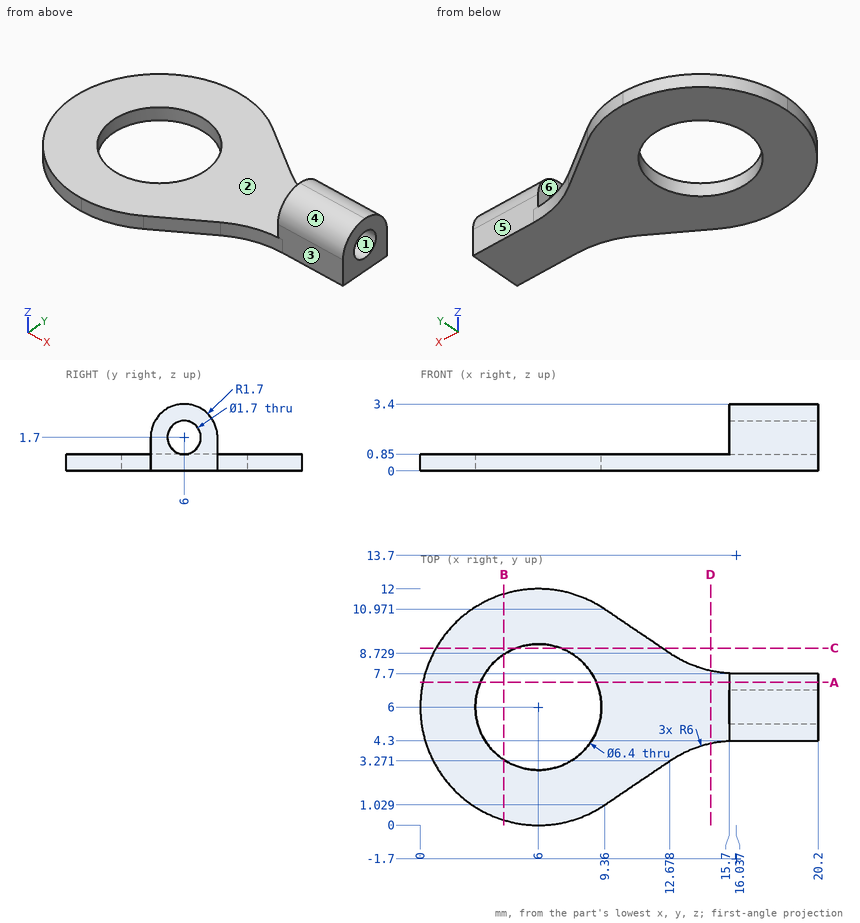
Here's the drawing with two shaded views (mm, measured from the low corner). I have some questions. A direction names the side the tool comes from. Round coordinates to 2 decimals unless told otherwise and drop trailing zeros. Loops run counter-clockwise (first coordinate to the right, second up) from the corner with the lowest first, then second, coordinate; pieces in that order, holes last. Notation, with made-up numbers: M 72.5,65 L 91.5,65 A18 cw 91.5,74 Z; hole C 16.25,53.5 d3. An arc over 180 degrees is marked long. Put each result on its own line as item: value.
Q1. Imagine slicing it at D-D (x = 14.75). Write out the boundary of the cut face in (y, z).
Check result:
outline: M 4.16,0 L 7.84,0 L 7.84,0.85 L 4.16,0.85 Z
Q2. Imagine slicing it at C-C (y = 9). Write out the boundary of the cut face in (x, z).
Check result:
outline: M 0.8,0 L 4.89,0 L 4.89,0.85 L 0.8,0.85 Z; M 7.11,0 L 12.28,0 L 12.28,0.85 L 7.11,0.85 Z
Q3. Imagine slicing it at A-A (y = 7.25). Write out the boundary of the cut face in (x, z).
Check result:
outline: M 0.13,0 L 3.05,0 L 3.05,0.85 L 0.13,0.85 Z; M 8.95,0 L 20.2,0 L 20.2,2.85 L 15.7,2.85 L 15.7,0.85 L 8.95,0.85 Z
Q4. I need wall thicknesses on probe 1 along Y at (x, z) = (6, 0.5); probe 2 along X at (y, z) = (6, 0.2); probe 3 along Z at (x, y) = (18.5, 6). Which ranges of each line are inside material? Lowest first, please.
Check result:
probe 1: 0 to 2.8, 9.2 to 12
probe 2: 0 to 2.8, 9.2 to 20.2
probe 3: 0 to 0.85, 2.55 to 3.4
Q5. For pin 1 (0.5 mm diameter, centred on x = 18.5, z = 1, fed in from +Y); pin 2 (1.4 mm diameter, centred on x = 17, z = 0.5, fed in from -Y); pin 3 (1 mm diameter, centred on y = 4.5, z = 3, fed in from -X), each with a flat end and sliding along its axis, tell me the tip position at first contact or that it passes through.
Check result:
pin 1: y = 7.7
pin 2: y = 4.3
pin 3: x = 15.7
Q6. Imagine slicing it at B-B (x = 4.25). Write out the boundary of the cut face in (y, z).
Check result:
outline: M 0.26,0 L 3.32,0 L 3.32,0.85 L 0.26,0.85 Z; M 8.68,0 L 11.74,0 L 11.74,0.85 L 8.68,0.85 Z
Q7. Thinking about a two-plate mould opening in Y: for the marked faces 1, 2 and 3, which applies, released by +Y, released by -Y, zero draft, split by the parting line, or undercut?
Check result:
face 1: undercut
face 2: zero draft
face 3: released by -Y
Q8. On a 3-axis mill with a long thin cutter (end or side, diameter ignored), from which of +Z, -Z, +X, -X, +Y, -Y can I reach the whole of each face in a straight line? I mean the marked faces 4, 5 and 6. Say none if no direction works.
Check result:
face 4: +Z, +X, -X, -Y
face 5: +Z, -Z, +X, +Y
face 6: +Z, -X, +Y, -Y
